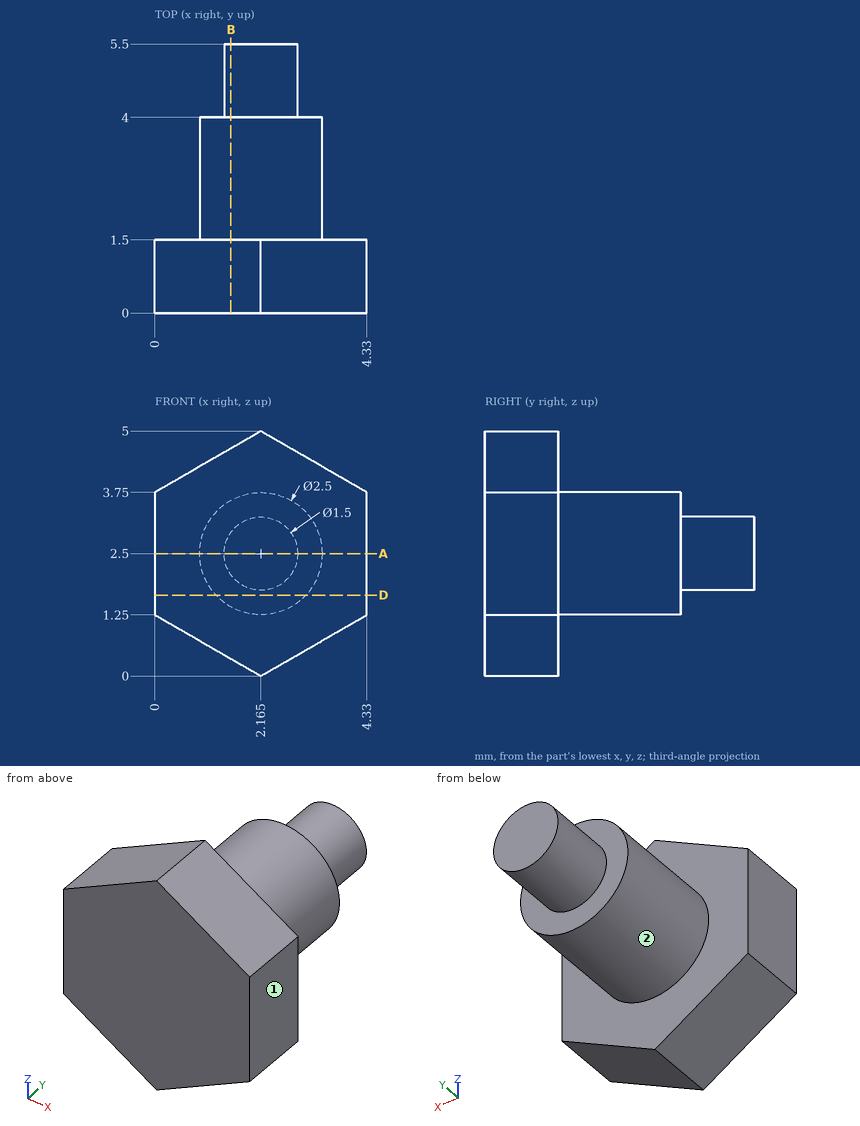
Design review of the part shown in the three views and the two pictorial views. Dimensions are in mm from the part's minimum x, y and z. A direction names the side the tool comes from. Round coordinates to 2 decimals unless told otherwise and drop trailing zeros. Write each loop counter-clockwise with the first axis right and the second up, starting at its lowest first coordinate (ties: lowest second). Pieces come first, ordered by that corner, then holes.
1) Take a section at A-A on z = 2.5. Give the boundary of the cut face in (x, y) (1 decimal), then the cut area to 3 significant figures.
Answer below:
outline: (0, 0) - (4.3, 0) - (4.3, 1.5) - (3.4, 1.5) - (3.4, 4) - (2.9, 4) - (2.9, 5.5) - (1.4, 5.5) - (1.4, 4) - (0.9, 4) - (0.9, 1.5) - (0, 1.5) - close
area: 15.0 mm2
2) Take a section at D-D on z = 1.65. Give the boundary of the cut face in (x, y), then the cut area to 3 significant figures.
Answer below:
outline: (0, 0) - (4.33, 0) - (4.33, 1.5) - (3.08, 1.5) - (3.08, 4) - (1.25, 4) - (1.25, 1.5) - (0, 1.5) - close
area: 11.1 mm2
3) Insertion check: pin 1 Ø2 at (x, y) = (3, 1) entering from +Z; pin 2 Ø1 at (x, y) = (1, 1.5) entering from +Z. Each pin has a flat end and moves straight along its axis. Give the tip position at first contact, or say it passes through.
Answer below:
pin 1: stops at z = 5
pin 2: stops at z = 4.62
4) For line 1 along Y through (x, z) = (2.85, 1.7); line 2 along Y through (x, z) = (3.8, 1.85); line 3 along X through (y, z) = (1.15, 4.75), list the stretches that pass through material, from the lowest coordinate up.
Answer below:
line 1: y = 0 to 4
line 2: y = 0 to 1.5
line 3: x = 1.73 to 2.6
5) Machinability: for the marked faces 1 and 2, which of the approach directions +Z, -Z, +X, -X, +Y, -Y give a long, thin tool a straight path to every point of the face, cutting with its end or side? Answer none if there is none.
Answer below:
face 1: +Z, -Z, +X, +Y, -Y
face 2: +Y
6) Take a section at B-B on x = 1.55. Give the boundary of the cut face in (y, z) (1 decimal).
Answer below:
outline: (0, 0.4) - (1.5, 0.4) - (1.5, 1.4) - (4, 1.4) - (4, 2.1) - (5.5, 2.1) - (5.5, 2.9) - (4, 2.9) - (4, 3.6) - (1.5, 3.6) - (1.5, 4.6) - (0, 4.6) - close
